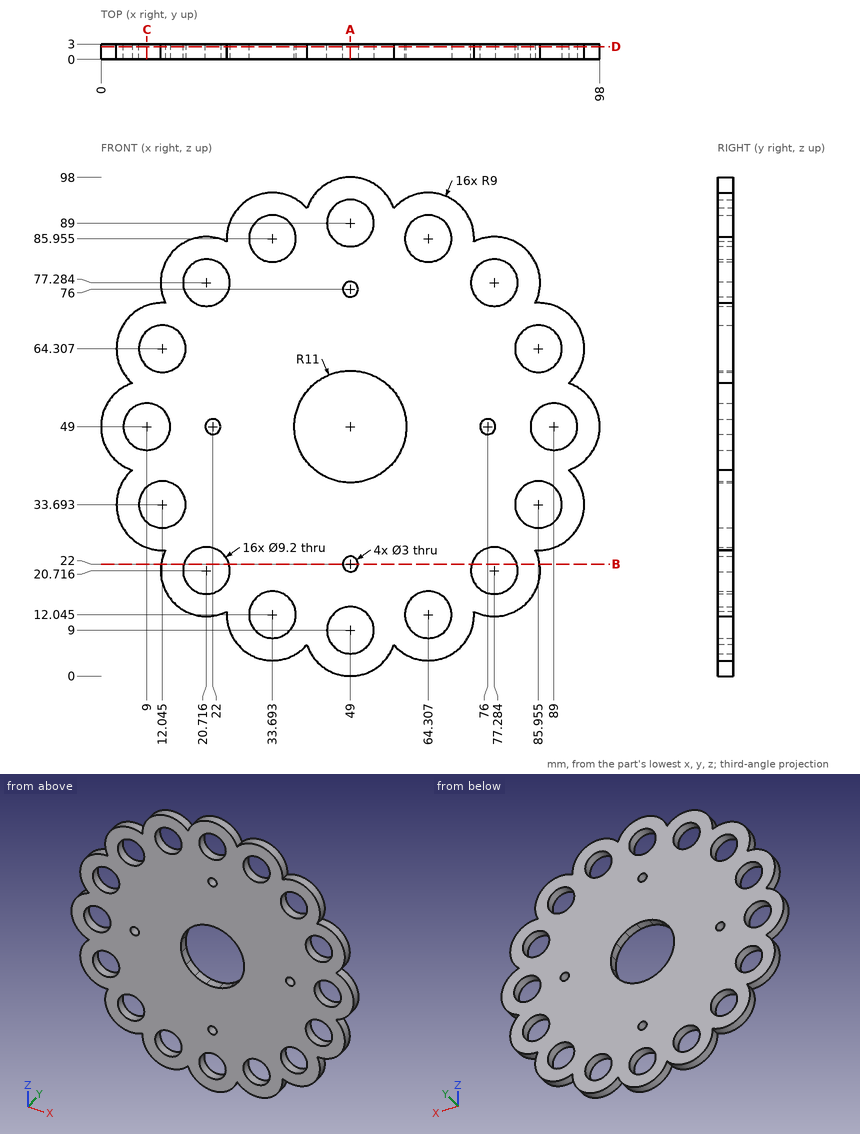
Answer from the drawing. Dimensions are ordinates in mm from the lowest x, y and z of the part. Round coordinates to 2 decimals unless told otherwise and drop trailing zeros. Loops run counter-clockwise (first coordinate to the right, second up) from the corner with the lowest first, then second, coordinate; pieces in that order, holes last.
1) Consider line 1 (X direction, y = 1.05, z = 64.5); line 2 (Z direction, x = 76, y = 2.1); line 3 (X direction, y = 0.55, z = 75.5) (1 decimal). Determine where each line is inside the solid, lowest interval first.
Outcome:
line 1: x = 3.05 to 7.45, 16.64 to 81.36, 90.55 to 94.95
line 2: z = 11.81 to 16.3, 25.13 to 47.5, 50.5 to 72.87, 81.7 to 86.19
line 3: x = 11.9 to 16.5, 25 to 47.6, 50.4 to 73, 81.5 to 86.1
2) A cutting plane is placed at D-D on y = 2.5. Give the number of separate pieces and of enclosed holes in the cut face, plus the area to 3 significant figures.
Outcome:
separate pieces: 1
enclosed holes: 21
area: 5,600 mm2
3) A cutting plane is placed at C-C on x = 9. Determine the outline of the cut face in (y, z) (1 decimal).
Outcome:
outline: (0, 25.2) - (3, 25.2) - (3, 30.2) - (0, 30.2) - close; (0, 37.1) - (3, 37.1) - (3, 44.4) - (0, 44.4) - close; (0, 53.6) - (3, 53.6) - (3, 60.9) - (0, 60.9) - close; (0, 67.8) - (3, 67.8) - (3, 72.8) - (0, 72.8) - close
4) Given P1, Ø2.5, axis at x = 22, z = 49, coming from the -Y side; P2, Ø1, axis at x = 39, y = 0.5, coming from the -Z side, each flat-ended and moving along its own axis, determine where each tip first touches the part or whether it passes through.
Outcome:
P1: passes through
P2: stops at z = 4.44
5) A cutting plane is placed at A-A on x = 49. Determine the outline of the cut face in (y, z), plus the area to 3 significant figures.
Outcome:
outline: (0, 0) - (3, 0) - (3, 4.4) - (0, 4.4) - close; (0, 13.6) - (3, 13.6) - (3, 20.5) - (0, 20.5) - close; (0, 23.5) - (3, 23.5) - (3, 38) - (0, 38) - close; (0, 60) - (3, 60) - (3, 74.5) - (0, 74.5) - close; (0, 77.5) - (3, 77.5) - (3, 84.4) - (0, 84.4) - close; (0, 93.6) - (3, 93.6) - (3, 98) - (0, 98) - close
area: 155 mm2
6) A cutting plane is placed at B-B on z = 22. Determine the outline of the cut face in (x, y), plus the area to 3 significant figures.
Outcome:
outline: (11.81, 0) - (16.3, 0) - (16.3, 3) - (11.81, 3) - close; (25.13, 0) - (47.5, 0) - (47.5, 3) - (25.13, 3) - close; (50.5, 0) - (72.87, 0) - (72.87, 3) - (50.5, 3) - close; (81.7, 0) - (86.19, 0) - (86.19, 3) - (81.7, 3) - close
area: 161 mm2
